Read the model definition and answer for the solid it produces. Units are mm, in the model's axes. Give positions to 0.01 mm unless a question says otherwise; leave off trailing zeros. Write each loop counter-clockwise with the first axis right and the second up, starting at its lowest first coordinate (ties: lowest second). Pieces come first, ordered by that corner, then holes. Notation, with made-up numbers: (29.5, 20.5) -> (42.5, 20.5) arc R18 cw to (42.5, 47.5) -> close; hole circle Ø1 at (7.25, -3.75). An arc over 180 degrees is marked (long way). Write item = value, one per line.
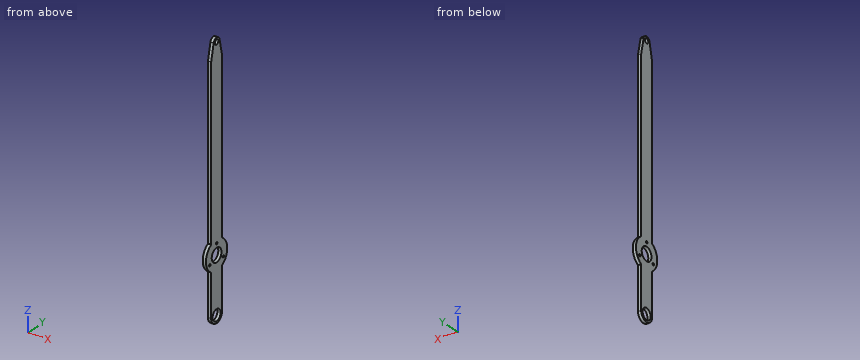
from build123d import *

# Parameters (mm, degrees)
SKETCH1_R            = 4.7625
SKETCH1_R_2          = 13.5
SKETCH1_R_3          = 11.1125
BOSS_EXTRUDE1_DEPTH  = 3.175
M4_CLEARANCE_HOLE1_D = 4.5


with BuildPart() as part:
    # Sketch1 → Boss-Extrude1 (new, symmetric)
    # profile 1 of 5: a face of its own
    with BuildSketch(Plane(origin=(0, 0, 0), x_dir=(0, 0, -1), z_dir=(1, 0, 0))):
        with BuildLine():
            Line((-135.401771592, 15), (-470, 15))
            Line((-470, 15), (-501.760727799, 8.072716015))
            ThreePointArc((-501.760727799, 8.072716015), (-508.2625, 0), (-501.760727799, -8.072716015))
            Line((-501.760727799, -8.072716015), (-470, -15))
            Line((-470, -15), (-135.401771592, -15))
            ThreePointArc((-135.401771592, -15), (-139.5, 0), (-135.401771592, 15))
        make_face()
        with Locations((-500, 0)):
            Circle(SKETCH1_R, mode=Mode.SUBTRACT)
    # profile 2 of 5: a face of its own
    with BuildSketch(Plane(origin=(0, 0, 0), x_dir=(0, 0, -1), z_dir=(1, 0, 0))):
        with BuildLine():
            Line((-84.598228408, -15), (-135.401771592, -15))
            ThreePointArc((-135.401771592, -15), (-110, -29.5), (-84.598228408, -15))
        make_face()
    # profile 3 of 5: a face of its own
    with BuildSketch(Plane(origin=(0, 0, 0), x_dir=(0, 0, -1), z_dir=(1, 0, 0))):
        with BuildLine():
            Line((-84.598228408, 15), (-135.401771592, 15))
            ThreePointArc((-135.401771592, 15), (-139.5, 0), (-135.401771592, -15))
            Line((-135.401771592, -15), (-84.598228408, -15))
            ThreePointArc((-84.598228408, -15), (-81.542995046, -7.774887075), (-80.5, 0))
            ThreePointArc((-80.5, 0), (-81.542995046, 7.774887075), (-84.598228408, 15))
        make_face()
        with Locations((-110, 0)):
            Circle(SKETCH1_R_2, mode=Mode.SUBTRACT)
    # profile 4 of 5: a face of its own
    with BuildSketch(Plane(origin=(0, 0, 0), x_dir=(0, 0, -1), z_dir=(1, 0, 0))):
        with BuildLine():
            ThreePointArc((-84.598228408, 15), (-110, 29.5), (-135.401771592, 15))
            Line((-135.401771592, 15), (-84.598228408, 15))
        make_face()
    # profile 5 of 5: a face of its own
    with BuildSketch(Plane(origin=(0, 0, 0), x_dir=(0, 0, -1), z_dir=(1, 0, 0))):
        with BuildLine():
            Line((0, 15), (-84.598228408, 15))
            ThreePointArc((-84.598228408, 15), (-81.542995046, 7.774887075), (-80.5, 0))
            ThreePointArc((-80.5, 0), (-81.542995046, -7.774887075), (-84.598228408, -15))
            Line((-84.598228408, -15), (0, -15))
            ThreePointArc((0, -15), (15, 0), (0, 15))
        make_face()
        Circle(SKETCH1_R_3, mode=Mode.SUBTRACT)
    extrude(amount=BOSS_EXTRUDE1_DEPTH, both=True)

    # M4 Clearance Hole1 (through all)
    with Locations(Plane(origin=(3.175, 0, 0), x_dir=(0, 0, -1), z_dir=(1, 0, 0))):
        with Locations((-110, 0), (-131.5, 0), (-99.25, 18.619546181), (-99.25, -18.619546181)):
            Hole(M4_CLEARANCE_HOLE1_D / 2)


solid = part.part
(1) The part is cut by section A-A on z = 110. Determine the outline of the cut face in (x, y) (3 decimals), plus the area to 3 significant figures.
Checks:
outline = (-3.175, -29.5) -> (3.175, -29.5) -> (3.175, -13.5) -> (-3.175, -13.5) -> close; (-3.175, 13.5) -> (3.175, 13.5) -> (3.175, 29.5) -> (-3.175, 29.5) -> close
area = 203 mm²
(2) The part is cut by section C-C on z = 272.5. Determine the outline of the cut face in (x, y) (3 decimals), plus the area to 4 significant figures.
Checks:
outline = (-3.175, -15) -> (3.175, -15) -> (3.175, 15) -> (-3.175, 15) -> close
area = 190.5 mm²
(3) Consider L1, parallel to Y at x = -0.25, z = 0; L2, parallel to Z at x = -0.5, y = 3; L3, parallel to Z at x = -2.5, y = -7.5. Determine where each line is inside the solid, lowest interval first.
Checks:
L1 = -15 to -11.11, 11.11 to 15
L2 = -14.7 to -10.7, 10.7 to 96.84, 123.16 to 496.3, 503.7 to 507.7
L3 = -12.99 to -8.2, 8.2 to 98.78, 121.22 to 503.47
(4) The part is cut by section B-B on x = -0.5. Count the separate pieces of the cut face and the enclosed holes in it, plus the area to 3 significant figures.
Checks:
separate_pieces = 1
enclosed_holes = 6
area = 15,200 mm²
(5) Given P1, Ø6, axis at y = 0, z = 131.5, coming from the -X side (3 decimals); P2, Ø3, axis at x = 0.5, z = 352, coming from the -Y side; P3, Ø1.5, axis at x = -2, y = 19.5, coming from the +Z side; P4, Ø1.9, axis at x = -1, z = 53.5, coming from the +Y side, each flat-ended and moving along its own axis, determine where each tip first touches the part or whether it passes through.
Checks:
P1 = -3.175
P2 = -15
P3 = 132.77
P4 = 15
